```python
from build123d import *

# Parameters (mm, degrees)
F0_R     = 12.7
F1_DEPTH = 50.8
F2_DEPTH = 19.05
F3_DEPTH = 22.352
F5_R     = 7.874
F5_R_2   = 3.2639
F7_DEPTH = 19.05


with BuildPart() as f1:
    # F0 (on Top) → F1 (new body)
    with BuildSketch(Plane.XY):
        with BuildLine():
            ThreePointArc((0, -22.225), (15.7154482119, -15.7154482119), (22.225, 0))
            ThreePointArc((22.225, 0), (15.7154482119, 15.7154482119), (0, 22.225))
            ThreePointArc((0, 22.225), (-22.225, 0), (0, -22.225))
        make_face()
        Circle(F0_R, mode=Mode.SUBTRACT)
    extrude(amount=F1_DEPTH)

    # F0 (on Top) → F2 (join)
    with BuildSketch(Plane.XY):
        with BuildLine():
            ThreePointArc((0, -22.225), (15.7154482119, -15.7154482119), (22.225, 0))
            ThreePointArc((22.225, 0), (15.7154482119, 15.7154482119), (0, 22.225))
            ThreePointArc((0, 22.225), (-22.225, 0), (0, -22.225))
        make_face()
        Circle(F0_R, mode=Mode.SUBTRACT)
        with BuildLine():
            ThreePointArc((0, -22.225), (-22.225, 0), (0, 22.225))
            Line((0, 22.225), (-20.2556934298, 22.225))
            ThreePointArc((-20.2556934298, 22.225), (-24.4127442388, 22.924627982), (-28.1117810213, 24.9464285714))
            ThreePointArc((-28.1117810213, 24.9464285714), (-37.3593729775, 30.0009300451), (-47.752, 31.75))
            Line((-47.752, 31.75), (-143.002, 31.75))
            ThreePointArc((-143.002, 31.75), (-174.752, 0), (-143.002, -31.75))
            Line((-143.002, -31.75), (-47.752, -31.75))
            ThreePointArc((-47.752, -31.75), (-37.3593729775, -30.0009300451), (-28.1117810213, -24.9464285714))
            ThreePointArc((-28.1117810213, -24.9464285714), (-24.4127442388, -22.924627982), (-20.2556934298, -22.225))
            Line((-20.2556934298, -22.225), (0, -22.225))
        make_face()
        with BuildLine():
            Line((-143.002, 19.05), (-47.752, 19.05))
            ThreePointArc((-47.752, 19.05), (-28.702, 0), (-47.752, -19.05))
            Line((-47.752, -19.05), (-143.002, -19.05))
            ThreePointArc((-143.002, -19.05), (-162.052, 0), (-143.002, 19.05))
        make_face(mode=Mode.SUBTRACT)
    extrude(amount=F2_DEPTH)

    # F0 (on Top) → F3 (join)
    with BuildSketch(Plane.XY):
        with BuildLine():
            ThreePointArc((-47.752, -19.05), (-28.702, 0), (-47.752, 19.05))
            Line((-47.752, 19.05), (-143.002, 19.05))
            ThreePointArc((-143.002, 19.05), (-162.052, 0), (-143.002, -19.05))
            Line((-143.002, -19.05), (-47.752, -19.05))
        make_face()
        with BuildLine():
            Line((-143.002, 9.525), (-47.752, 9.525))
            ThreePointArc((-47.752, 9.525), (-38.227, 0), (-47.752, -9.525))
            Line((-47.752, -9.525), (-143.002, -9.525))
            ThreePointArc((-143.002, -9.525), (-152.527, 0), (-143.002, 9.525))
        make_face(mode=Mode.SUBTRACT)
    extrude(amount=F3_DEPTH)

    # F5 (on offset) → F6 (join, up to the next surface of F1)
    with BuildSketch(Plane.YZ.offset(25.4)):
        with Locations((0, 31.75)):
            Circle(F5_R)
        with Locations((0, 31.75)):
            Circle(F5_R_2, mode=Mode.SUBTRACT)
    extrude(until=Until.NEXT, dir=(-1, 0, 0))

    # F5 (on offset) → F7 (cut)
    with BuildSketch(Plane.YZ.offset(25.4)):
        with Locations((0, 31.75)):
            Circle(F5_R_2)
    extrude(amount=-F7_DEPTH, mode=Mode.SUBTRACT)


solid = f1.part
```
Can you work these out from the model? Positions are in its coordinate system, mm. A direction names the side the tool comes from. Give positions to 0.01 mm unless a question says otherwise; leave off trailing zeros. Loops run counter-clockwise (first coordinate to the right, second up) from the corner with the lowest first, then second, coordinate; pieces in that order, holes last. Notation, with made-up numbers: M 73.25,67.5 L 122.25,67.5 A23 ccw 122.25,87.5 Z; hole C 39,-14 d5. An arc over 180 degrees is marked long. Use one line per item in the form item = value. Start each with the question number.
(1) On a 3-axis mill with a long thin cutter (end or side, diameter ignored), from which of +Z, -Z, +X, -X, +Y, -Y can I reach the whole of each face in a straight line? I mean faces 4 (the flat face through (-10, 22.225, 9)), 5 (the flat face through (-96, 9.525, 11)), 6 (the flat face through (-10, -22.225, 9)), 7 (the cylindrical face through (-162.047, 0.419, 20.678)). Say none if no direction works.
(2) I'm going to push flat-ended pins straight in: P1, Ø21, axis at x = -9, z = 9.5, coming from the -Y side (3 decimals); P2, Ø4, axis at y = -5, z = 13.5, coming from the -X side; P3, Ø12, axis at y = -2, z = 7, coming from the -X side; P4, Ø1, axis at x = -96, z = 24.5, coming from the +Y side. Where does each tip first touch, or does it pass through?
(3) Please list where these lines run through material, in increasing order: line 1 (Y direction, x = 24.05, z = 31.75); line 2 (Z direction, x = 24, y = 0); line 3 (Y direction, x = -91, z = 6) (3 decimals).
(4) Thinking about a two-plate mould opening in X: for faces 1 (the cylindrical face through (-152.525, -0.209, 11.02)), 2 (the flat face through (-96, 13, 22.352)), 3 (the cylindrical face through (-24.469, -22.944, 9.392)), which applies, released by +X, released by -X, zero draft, split by the parting line, or undercut?
(5) I want a section at D-D, the plane y = 15. Write out the boundary of the cut face in (x, z), and give its area (3 significant figures).
(6) I want a section at C-C, the plane z = 31.75. Write out the boundary of the cut face in (x, y) (3 decimals).
(7) I want a section at B-B, the plane x = -109.5. Write out the boundary of the cut face in (y, z) (3 decimals).
(8) I want a section at A-A, the plane z = 5. Write out the boundary of the cut face in (x, y) (3 decimals).
Worked out:
q1.face_4 = +Z, -Z, +X, +Y
q1.face_5 = +Z, -Z
q1.face_6 = +Z, -Z, +X, -Y
q1.face_7 = +Z, -X
q2.P1 = -22.225
q2.P2 = -174.61
q2.P3 = -174.75
q2.P4 = through
q3.line_1 = -7.87 to -3.26, 3.26 to 7.87
q3.line_2 = 23.88 to 28.49, 35.01 to 39.62
q3.line_3 = -31.75 to -9.525, 9.525 to 31.75
q4.face_1 = undercut
q4.face_2 = zero draft
q4.face_3 = released by +X
q5.outline = M -170.99,0 L 16.4,0 L 16.4,50.8 L -16.4,50.8 L -16.4,19.05 L -36.01,19.05 L -36.01,22.35 L -154.75,22.35 L -154.75,19.05 L -170.99,19.05 Z
q5.area = 5,000 mm²
q6.outline = M 12.273,-3.264 A12.7 cw long 12.273,3.264 L 25.4,3.264 L 25.4,7.874 L 20.783,7.874 A22.225 ccw long 20.783,-7.874 L 25.4,-7.874 L 25.4,-3.264 Z
q7.outline = M -31.75,0 L -9.525,0 L -9.525,22.352 L -19.05,22.352 L -19.05,19.05 L -31.75,19.05 Z; M 9.525,0 L 31.75,0 L 31.75,19.05 L 19.05,19.05 L 19.05,22.352 L 9.525,22.352 Z
q8.outline = M -143.002,-31.75 L -47.752,-31.75 A31.75 ccw -28.112,-24.946 A12.7 cw -20.256,-22.225 L 0,-22.225 A22.225 ccw 0,22.225 L -20.256,22.225 A12.7 cw -28.112,24.946 A31.75 ccw -47.752,31.75 L -143.002,31.75 A31.75 ccw Z; hole M -143.002,-9.525 L -47.752,-9.525 A9.525 ccw -47.752,9.525 L -143.002,9.525 A9.525 ccw Z; hole C 0,0 d25.4
